Verification items for the finished model (mm, model axes). A direction names the side the tool comes from. Coordinates: 2 decimals unless noted, no trailing zeros. Loops run counter-clockwise (first coordinate to the right, second up) from the corner with the lowest first, then second, coordinate; pieces in that order, holes last. Notation, with made-up numbers: (-32, -9.5) - (-27, -9.5) arc R25 cw to (-27, 13.5) - close; hole circle Ø9 at (72, 70.25). An arc over 180 degrees is marked (long way). Answer as CSV lines item,"result". Start each with the question number.
1. Gauge pin test, flat ends, axial feed: P1, Ø4, axis at x = 19, z = 55.5, coming from the -Y side; P2, Ø3, axis at x = 21, y = 28.5, coming from the +Z side; P3, Ø6.5, axis at y = 46, z = 6, coming from the +X side. Record the tip position at first contact, or that the pin passes through.
2. Cross-section at A-A (z = 31). Enter the section's corners in (x, y), plus the area to 3 significant figures.
3. Release check for a two-part mould opening along Y. For faces 1 (the flat face through (3.77, 38.42, 22.68)), 2 (the flat face through (21, 0, 23)), 3 (the cylindrical face through (5.325, 35.186, 43.782)), 4 (the flat face through (37, 6, 41.5)) record: pulls with the +Y half, pulls with the -Y half, needs draft (parallel to the pull), parting line crosses it, or undercut.
4. Cross-section at C-C (y = 5.65). Enter the section's corners in (x, z), plus the area to 3 significant figures.
5. Set-up check for faces 5 (the flat face through (12, 12, 46)), 6 (the flat face through (13.65, 45, 5)), 7 (the flat face through (21, 45, 10)): record each of +Z, -Z, +X, -X, +Y, -Y from which the full face is reachable in a straight line by a thin tool's end or side.
6. Cross-section at B-B (z = 44). Enter the section's corners in (x, y).
7. Material ranges on line 1 (Y direction, x = 36.65, z = 44.1); line 2 (X direction, y = 36, z = 44); line 3 (Y direction, x = 5, z = 44), recorded low to high. Write a range as [from, to].
```python
from build123d import *

# Parameters (mm, degrees)
BOSS_EXTRUDE1_DEPTH = 46
SKETCH3_R           = 11
BOSS_EXTRUDE2_DEPTH = 2
SKETCH4_R           = 2.5
BOSS_EXTRUDE3_DEPTH = 22
CUT_EXTRUDE1_START  = -22
CUT_EXTRUDE1_DEPTH  = 22
SKETCH6_R           = 1.5
CUT_EXTRUDE2_DEPTH  = 4.5
SKETCH7_W           = 15
SKETCH7_H           = 10
BOSS_EXTRUDE4_DEPTH = 6


with BuildPart() as part:
    # Sketch1 → Boss-Extrude1 (new body)
    with BuildSketch(Plane.XY):
        Polygon((7.65, 0), (0, 7.65), (0, 34.65), (7.65, 42.3), (34.65, 42.3), (42.3, 34.65), (42.3, 7.65), (34.65, 0), align=None)
    extrude(amount=BOSS_EXTRUDE1_DEPTH)

    # Sketch3 → Boss-Extrude2 (add)
    with BuildSketch(Plane.XY.offset(46)):
        with Locations((21.15, 21.15)):
            Circle(SKETCH3_R)
    extrude(amount=BOSS_EXTRUDE2_DEPTH)

    # Sketch4 → Boss-Extrude3 (add)
    with BuildSketch(Plane.XY.offset(48)):
        with Locations((21.15, 21.15)):
            Circle(SKETCH4_R)
    extrude(amount=BOSS_EXTRUDE3_DEPTH)

    # Sketch5 → Cut-Extrude1 (cut)
    with BuildSketch(Plane.XY.offset(70).offset(CUT_EXTRUDE1_START)):
        with BuildLine():
            Line((21.15, 23.15), (22.65, 23.15))
            ThreePointArc((22.65, 23.15), (21.15, 23.65), (19.65, 23.15))
            Line((19.65, 23.15), (21.15, 23.15))
        make_face()
    extrude(amount=CUT_EXTRUDE1_DEPTH, mode=Mode.SUBTRACT)

    # Sketch6 → Cut-Extrude2 (cut)
    with BuildSketch(Plane.XY.offset(46)):
        with Locations((5.65, 5.65)):
            Circle(SKETCH6_R)
        with Locations((5.65, 36.65)):
            Circle(SKETCH6_R)
        with Locations(Location((36.65, 5.65, 0), (0, 0, 180))):
            Circle(SKETCH6_R)
        with Locations(Location((36.65, 36.65, 0), (0, 0, 180))):
            Circle(SKETCH6_R)
    extrude(amount=-CUT_EXTRUDE2_DEPTH, mode=Mode.SUBTRACT)

    # Sketch7 → Boss-Extrude4 (add)
    with BuildSketch(Plane(origin=(0, 42.3, 0), x_dir=(1, 0, 0), z_dir=(0, 1, 0))):
        with Locations((21.15, -5)):
            Rectangle(SKETCH7_W, SKETCH7_H)
    extrude(amount=BOSS_EXTRUDE4_DEPTH)


solid = part.part
```
Values follow:
1,P1,"stops at y = 18.65"
1,P2,"stops at z = 48"
1,P3,"stops at x = 28.65"
2,outline,"(0, 7.65) - (7.65, 0) - (34.65, 0) - (42.3, 7.65) - (42.3, 34.65) - (34.65, 42.3) - (7.65, 42.3) - (0, 34.65) - close"
2,area,"1,670 mm²"
3,face 1,"pulls with the +Y half"
3,face 2,"pulls with the -Y half"
3,face 3,"undercut"
3,face 4,"undercut"
4,outline,"(2, 0) - (40.3, 0) - (40.3, 46) - (38.15, 46) - (38.15, 41.5) - (35.15, 41.5) - (35.15, 46) - (7.15, 46) - (7.15, 41.5) - (4.15, 41.5) - (4.15, 46) - (2, 46) - close"
4,area,"1,730 mm²"
5,face 5,"+Z"
5,face 6,"+Z, -Z, -X, +Y"
5,face 7,"+Z, +X, -X, +Y"
6,outline,"(0, 7.65) - (7.65, 0) - (34.65, 0) - (42.3, 7.65) - (42.3, 34.65) - (34.65, 42.3) - (7.65, 42.3) - (0, 34.65) - close; hole circle Ø3 at (5.65, 5.65); hole circle Ø3 at (5.65, 36.65); hole circle Ø3 at (36.65, 5.65); hole circle Ø3 at (36.65, 36.65)"
7,line 1,"y = [2, 4.15], [7.15, 35.15], [38.15, 40.3]"
7,line 2,"x = [1.35, 4.3], [7, 35.3], [38, 40.95]"
7,line 3,"y = [2.65, 4.3], [7, 35.3], [38, 39.65]"
